Here's how the part is built. I have some questions about the finished solid (model axes, mm). Face numbers are marked on the shaded views. A direction names the side the tool comes from. Round coordinates to 2 decimals unless told otherwise and drop trailing zeros. Loops run counter-clockwise (first coordinate to the right, second up) from the corner with the lowest first, then second, coordinate; pieces in that order, holes last. Notation, with made-up numbers: M 14,-11 L 31,-11 A26 cw 31,11 Z; hole C -17,25.25 d1. An arc over 180 degrees is marked long. One line per question, with ' | ' between items. Start each with the question number.
```python
from build123d import *

# Parameters (mm, degrees)
F1_DEPTH      = 2.1
F1_DEPTH_BACK = 1.8
F2_R          = 1.75
F3_DEPTH      = 3.3
F4_W          = 6.85
F4_H          = 7.9
F5_DEPTH      = 4
F6_W          = 8
F6_H          = 2.1
F7_DEPTH      = 4


with BuildPart() as f1:
    # F0 (on Top) → F1 (new body, two sides)
    with BuildSketch(Plane.XY) as f1_sk:
        Polygon((10, -8.5), (10, 8.5), (3.75, 8.5), (3.75, 13.5), (-2, 13.5), (-2, 8.5), (-10, 8.5), (-10, -8.5), align=None)
    extrude(amount=F1_DEPTH)
    extrude(f1_sk.sketch, amount=-F1_DEPTH_BACK)

    # F2 (on Top) → F3 (join)
    with BuildSketch(Plane.XY):
        with Locations((0.875, 11)):
            Circle(F2_R)
    extrude(amount=F3_DEPTH)

    # F4 (on Top) → F5 (join)
    with BuildSketch(Plane.XY):
        with Locations((-6.075, 3.8)):
            Rectangle(F4_W, F4_H)
    extrude(amount=F5_DEPTH)

    # F6 (on face) → F7 (join)
    with BuildSketch(Plane.XZ.offset(8.5)):
        with Locations((6, 1.05)):
            Rectangle(F6_W, F6_H)
    extrude(amount=F7_DEPTH)


solid = f1.part
```
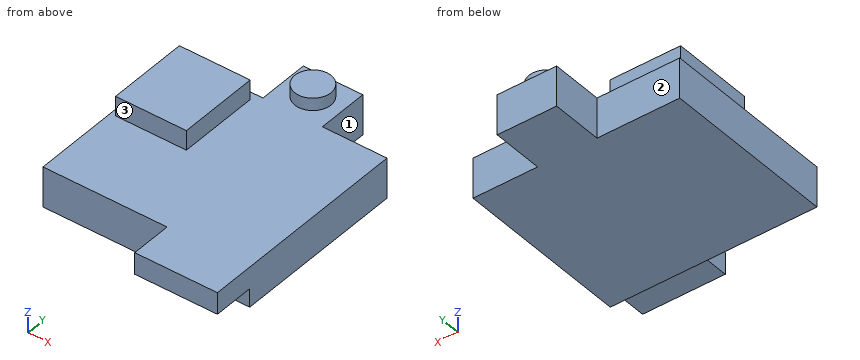
1) For the marked faces 1, 2 and 3, which set-ups out of +Z, -Z, +X, -X, +Y, -Y let a thin tool reach every point of the face, with its end or its side?
2) Please list where these lines run through material, in increasing order: L1, parallel to Y at x = -8, z = -0.75; L2, parallel to Z at x = -6.5, y = -5.5; L3, parallel to Y at x = -3.75, z = 2.3. Write a range as from..to.
3) Imagine slicing it at B-B (x = 3). Write out the boundary of the cut face in (y, z), then the cut area to 3 significant figures.
4) Imagine slicing it at D-D (z = -1). Write out the boundary of the cut face in (x, y), then the cut area to 3 significant figures.
5) Imagine slicing it at C-C (y = 1.5). Write out the boundary of the cut face in (x, z), then the cut area to 3 significant figures.
6) Imagine slicing it at A-A (z = 2.5). Write out the boundary of the cut face in (x, y) (3 decimals).
7) I'm going to push flat-ended pins straight in: pin 1 Ø1.5 at (x, z) = (-7, 3) entering from +Y; pin 2 Ø0.6 at (y, z) = (5.5, 3) entering from +X; pin 3 Ø1.2 at (y, z) = (12, 0.5) entering from -X. Where does each tip first touch, or does it pass through?
Results are:
1) face 1: +Z, -Z, +X, +Y | face 2: +Z, -Z, -X, +Y | face 3: +Z, +X, -X, -Y
2) L1: -8.5..8.5 | L2: -1.8..2.1 | L3: -0.15..7.75
3) outline: M -12.5,0 L -8.5,0 L -8.5,-1.8 L 13.5,-1.8 L 13.5,2.1 L -12.5,2.1 Z | area: 94.2 mm²
4) outline: M -10,-8.5 L 10,-8.5 L 10,8.5 L 3.75,8.5 L 3.75,13.5 L -2,13.5 L -2,8.5 L -10,8.5 Z | area: 369 mm²
5) outline: M -10,-1.8 L 10,-1.8 L 10,2.1 L -2.65,2.1 L -2.65,4 L -9.5,4 L -9.5,2.1 L -10,2.1 Z | area: 91.0 mm²
6) outline: M -9.5,-0.15 L -2.65,-0.15 L -2.65,7.75 L -9.5,7.75 Z; C 0.875,11 d3.5
7) pin 1: y = 7.75 | pin 2: x = -2.65 | pin 3: x = -2
